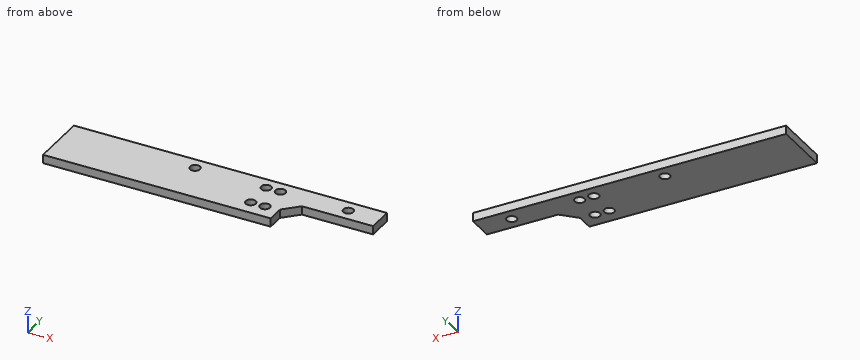
Autodesk Inventor part; units mm, degrees
ref_plane "YZ Plane" through (0, 0, 0) normal (1, 0, 0) x (0, 1, 0)
ref_plane "XZ Plane" through (0, 0, 0) normal (0, 1, 0) x (-1, 0, 0)
ref_plane "XY Plane" through (0, 0, 0) normal (0, 0, 1) x (1, 0, 0)
sketch "Sketch1" plane through (0, 0, 0) normal (0, 0, 1) x (1, 0, 0)
  line L0 (76.2, -5.715) -> (-76.2, -5.715)
  line L1 (-76.2, -5.715) -> (-76.2, 5.715)
  line L2 (-76.2, 5.715) -> (76.2, 5.715)
  line L3 (76.2, 5.715) -> (76.2, -5.715)
  line L4 (76.2, -5.715) -> (-76.2, 5.715) construction
  line L5 (-76.2, -5.715) -> (76.2, 5.715) construction
  circle A0 centre (-6.35, 0) radius 2.25
  circle A1 centre (62.0522, 0) radius 2.25
  circle A2 centre (25.4, 0) radius 2.25
  circle A3 centre (31.75, 0) radius 2.25
  circle A4 centre (25.4, -12.7) radius 2.25
  circle A5 centre (31.75, -12.7) radius 2.25
  line L6 (0, 5.715) -> (-76.2, 5.715)
  line L7 (38.1, 5.715) -> (-63.5, 5.715)
  line L8 (-63.5, 5.715) -> (-63.5, -19.685)
  line L9 (-63.5, -19.685) -> (38.1, -19.685)
  line L10 (38.1, -19.685) -> (38.1, 5.715)
  point P0 (0, 0)
  point P1 (38.1, -5.715)
  point P2 (-63.5, -5.715)
  dimension "d0" = 152.4
  dimension "d1" = 11.43
  dimension "d2" = 4.5
  dimension "d3" = 4.5
  dimension "d4" = 68.4022
  dimension "d5" = 69.85
  dimension "d6" = 4.5
  dimension "d9" = 101.6
  dimension "d12" = 6.35
  dimension "d15" = 12.7
  dimension "d22" = 101.6
  dimension "d23" = 25.4
  dimension "d24" = 6.35
extrude "Extrusion1" add sketch "Sketch1" along normal blind 3.81
fillet "Fillet1" [suppressed]
sketch "Sketch2" plane through (0, 0, 3.81) normal (0, 0, 1) x (1, 0, 0)
  line L0 (76.2, 5.715) -> (-76.2, 5.715)
  line L1 (-76.2, 5.715) -> (-76.2, -5.715)
  line L2 (-76.2, -5.715) -> (-63.5, -5.715)
  line L3 (-63.5, -5.715) -> (-63.5, -19.685)
  line L4 (-63.5, -19.685) -> (38.1, -19.685)
  line L5 (38.1, -19.685) -> (38.1, -5.715)
  line L6 (38.1, -5.715) -> (76.2, -5.715)
  line L7 (76.2, -5.715) -> (76.2, 5.715)
  circle A0 centre (-6.35, 0) radius 2.25
  circle A1 centre (62.0522, 0) radius 2.25
  circle A2 centre (25.4, 0) radius 2.25
  circle A3 centre (31.75, 0) radius 2.25
  circle A4 centre (31.75, -12.7) radius 2.25
  circle A5 centre (25.4, -12.7) radius 2.25
  line L8 (-63.5, -5.715) -> (-76.2, -5.715)
  line L9 (-76.2, -5.715) -> (-76.2, 5.715)
  line L10 (-76.2, 5.715) -> (-63.5, 5.715)
  line L11 (-63.5, 5.715) -> (-63.5, -5.715)
  point P0 (0, 0)
extrude "Extrusion2" cut sketch "Sketch2" against normal through all contours L11 L2 L1 L0
chamfer "Chamfer1" distance 6.35 angle 45 1 edges at (38.1, -5.715, 1.905)
properties part number "Slide_Climb_Hook_Mounts"
Verification items for the finished model (mm, model axes). Give positions to 0.01 mm unless a question says otherwise; leave off trailing zeros. Order: outer loops, then holes, each group sorted by start corner. A loop starts at its lowest first (then second) coordinate and runs counter-clockwise, first axis right, second up. Notation, with made-up numbers: (62, -36) -> (86, -36) arc R21 ccw to (86, -30) -> close; hole circle Ø6 at (63, 87.25). An arc over 180 degrees is marked (long way). One line per item, written item: value.
(1) Gauge pin test, flat ends, axial feed: pin 1 (5 mm diameter, centred on x = 25.4, y = -12.7, fed in from +Z); pin 2 (1.1 mm diameter, centred on y = -16, z = 2, fed in from +X); pin 3 (1.1 mm diameter, centred on x = 66.5, z = 2, fed in from -Y) (3 decimals). Record the tip position at first contact, or that the pin passes through.
Final values:
pin 1: z = 3.81
pin 2: x = 38.1
pin 3: y = -5.715
(2) Sectioned sample at B-B on z = 2.1. Record the cut outline in (x, y) (3 decimals).
Final values:
outline: (-63.5, -19.685) -> (38.1, -19.685) -> (38.1, -12.065) -> (44.45, -5.715) -> (76.2, -5.715) -> (76.2, 5.715) -> (-63.5, 5.715) -> close; hole circle Ø4.5 at (-6.35, 0); hole circle Ø4.5 at (25.4, -12.7); hole circle Ø4.5 at (25.4, 0); hole circle Ø4.5 at (31.75, -12.7); hole circle Ø4.5 at (31.75, 0); hole circle Ø4.5 at (62.052, 0)
(3) Scan lines: line 1 along Y through (x, z) = (31.75, 2.5) (3 decimals); line 2 along X through (y, z) = (-11.5, 1.65) (3 decimals); line 3 along Y through (x, z) = (58.5, 3.5) (3 decimals). Record each from-to range of solid material in increasing order. Write a range as [from, to].
Final values:
line 1: [-19.685, -14.95], [-10.45, -2.25], [2.25, 5.715]
line 2: [-63.5, 23.497], [27.303, 29.847], [33.653, 38.665]
line 3: [-5.715, 5.715]
(4) Sectioned sample at D-D on x = 57.5. Record the cut outline in (y, z) (3 decimals), then the cut area to 3 significant figures.
Final values:
outline: (-5.715, 0) -> (5.715, 0) -> (5.715, 3.81) -> (-5.715, 3.81) -> close
area: 43.5 mm^2
(5) Sectioned sample at A-A on y = 0. Record the cut outline in (x, z), then the cut area to 3 significant figures.
Final values:
outline: (-63.5, 0) -> (-8.6, 0) -> (-8.6, 3.81) -> (-63.5, 3.81) -> close; (-4.1, 0) -> (23.15, 0) -> (23.15, 3.81) -> (-4.1, 3.81) -> close; (27.65, 0) -> (29.5, 0) -> (29.5, 3.81) -> (27.65, 3.81) -> close; (34, 0) -> (59.8, 0) -> (59.8, 3.81) -> (34, 3.81) -> close; (64.3, 0) -> (76.2, 0) -> (76.2, 3.81) -> (64.3, 3.81) -> close
area: 464 mm^2
(6) Sectioned sample at C-C on x = 31.75. Record the cut outline in (y, z) (3 decimals).
Final values:
outline: (-19.685, 0) -> (-14.95, 0) -> (-14.95, 3.81) -> (-19.685, 3.81) -> close; (-10.45, 0) -> (-2.25, 0) -> (-2.25, 3.81) -> (-10.45, 3.81) -> close; (2.25, 0) -> (5.715, 0) -> (5.715, 3.81) -> (2.25, 3.81) -> close
